Answer from the drawing. Dimensions are ordinates in mm from the lowest x, y and z of the part. Coordinates: 2 decimals unless noted, no trailing zeros. Write each loop counter-clockwise with the first axis right and the second up, starting at its lowest first coordinate (ties: lowest second). Pieces come first, ordered by that corner, then holes.
(1) Given pin 1 (1.8 mm diameter, centred on y = 3, z = 13, fed in from +X); pin 2 (4 mm diameter, centred on y = 3, z = 25.5, fed in from -X); pin 3 (10 mm diameter, centred on x = 39, z = 12, fed in from +Y); pin 4 (12 mm diameter, centred on x = 31, z = 13, fed in from +Y), each flat-ended and moving along its own axis, determine where each tip first touches the part or whether it passes through.
(2) The part is cut by section A-A, the plane y = 2.5. Determine the outline of the cut face in (x, z).
(3) The part is cut by section B-B, the plane z = 21.5. Determine the outline of the cut face in (x, y).
(4) The part is cut by section C-C, the plane x = 6.5. Determine the outline of the cut face in (y, z).
(5) The part is cut by section D-D, the plane z = 6.5. Determine the outline of the cut face in (x, y), and give its area (3 significant figures).
(6) Straight lines are drawn through the part: line 1 along X through (y, z) = (2, 20); line 2 along X through (y, z) = (4.5, 32); line 3 along Y through (x, z) = (57, 33). For each, find the intervals that lie inside material, in ascending order.
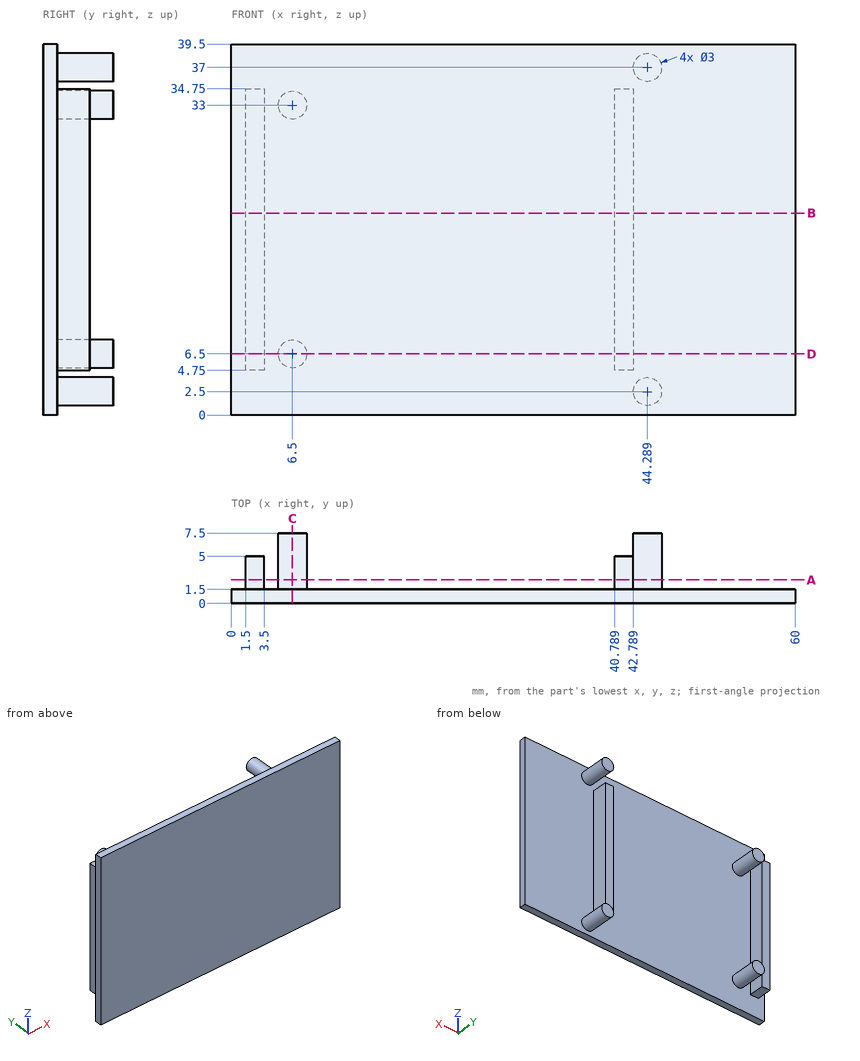
Computed:
1. pin 1: stops at x = 42.79
1. pin 2: stops at x = 0
1. pin 3: stops at y = 5
1. pin 4: stops at y = 1.5
2. outline: (1.5, 4.75) - (3.5, 4.75) - (3.5, 34.75) - (1.5, 34.75) - close; circle Ø3 at (6.5, 6.5); circle Ø3 at (6.5, 33); (40.79, 4.75) - (42.79, 4.75) - (42.79, 34.75) - (40.79, 34.75) - close; circle Ø3 at (44.29, 2.5); circle Ø3 at (44.29, 37)
3. outline: (0, 0) - (60, 0) - (60, 1.5) - (42.79, 1.5) - (42.79, 5) - (40.79, 5) - (40.79, 1.5) - (3.5, 1.5) - (3.5, 5) - (1.5, 5) - (1.5, 1.5) - (0, 1.5) - close
4. outline: (0, 0) - (1.5, 0) - (1.5, 5) - (7.5, 5) - (7.5, 8) - (1.5, 8) - (1.5, 31.5) - (7.5, 31.5) - (7.5, 34.5) - (1.5, 34.5) - (1.5, 39.5) - (0, 39.5) - close
5. outline: (0, 0) - (60, 0) - (60, 1.5) - (42.79, 1.5) - (42.79, 5) - (40.79, 5) - (40.79, 1.5) - (8, 1.5) - (8, 7.5) - (5, 7.5) - (5, 1.5) - (3.5, 1.5) - (3.5, 5) - (1.5, 5) - (1.5, 1.5) - (0, 1.5) - close
5. area: 122 mm2
6. line 1: x = 1.5 to 3.5, 40.79 to 42.79
6. line 2: x = 1.5 to 3.5, 5.38 to 7.62, 40.79 to 42.79
6. line 3: y = 0 to 1.5
